Check sheet for the modelled part. Datum: model origin and axes. Units: mm. A direction names the side the tool comes from. Round coordinates to 2 decimals unless told otherwise and drop trailing zeros. Write each loop counter-clockwise with the first axis right and the second up, starting at its lowest first coordinate (ties: lowest second). Pieces come first, ordered by that corner, then holes. Notation, with made-up numbers: (82, 4.5) -> (93, 4.5) arc R19 ccw to (93, 17.5) -> close; hole circle Ø8 at (30.25, 42). An arc over 180 degrees is marked (long way). One line per item, written item: value.
from build123d import *

# Parameters (mm, degrees)
BOSS_EXTRUDE1_DEPTH = 5
SKETCH3_R           = 10.5
CUT_EXTRUDE1_DEPTH  = 1
SKETCH4_R           = 2.5
BOSS_EXTRUDE2_DEPTH = 6
SKETCH5_R           = 1.5
CUT_EXTRUDE2_DEPTH  = 3
CUT_EXTRUDE3_DEPTH  = 1
SKETCH7_R           = 1.25
CUT_EXTRUDE4_DEPTH  = 5
SKETCH8_R           = 2.5
CUT_EXTRUDE5_DEPTH  = 0.5
CUT_EXTRUDE6_DEPTH  = 2
CUT_EXTRUDE7_DEPTH  = 2
SKETCH12_R          = 12.1
BOSS_EXTRUDE3_DEPTH = 15
SKETCH13_R          = 10.4
SKETCH13_R_2        = 2.5
CUT_EXTRUDE8_DEPTH  = 14
SKETCH14_R          = 1.5
CUT_EXTRUDE9_DEPTH  = 5


with BuildPart() as part:
    # Sketch1 → Boss-Extrude1 (new body)
    with BuildSketch(Plane(origin=(0, 0, 0), x_dir=(1, 0, 0), z_dir=(0, 1, 0))):
        with BuildLine():
            Line((-22, -23.004932369), (-22, -33.004932369))
            Line((-22, -33.004932369), (-13.5, -33.004932369))
            Line((-13.5, -33.004932369), (-8.890227771, -30.004932369))
            Line((-8.890227771, -30.004932369), (-7.526591408, -32.100283382))
            ThreePointArc((-7.526591408, -32.100283382), (-3.847417482, -30.904492858), (0, -30.5))
            Line((0, -30.5), (0, 12.5))
            ThreePointArc((0, 12.5), (-7.116131574, 10.276705281), (-11.700861907, 4.397707428))
            Line((-11.700861907, 4.397707428), (-22, -23.004932369))
        make_face()
        with BuildLine():
            ThreePointArc((11.700861907, 4.397707428), (7.116131574, 10.276705281), (0, 12.5))
            Line((0, 12.5), (0, -30.5))
            ThreePointArc((0, -30.5), (3.847417482, -30.904492858), (7.526591408, -32.100283382))
            Line((7.526591408, -32.100283382), (8.890227771, -30.004932369))
            Line((8.890227771, -30.004932369), (13.5, -33.004932369))
            Line((13.5, -33.004932369), (22, -33.004932369))
            Line((22, -33.004932369), (22, -23.004932369))
            Line((22, -23.004932369), (11.700861907, 4.397707428))
        make_face()
    extrude(amount=BOSS_EXTRUDE1_DEPTH)

    # Sketch3 → Cut-Extrude1 (cut)
    with BuildSketch(Plane(origin=(0, 5, 0), x_dir=(1, 0, 0), z_dir=(0, 1, 0))):
        Circle(SKETCH3_R)
    extrude(amount=-CUT_EXTRUDE1_DEPTH, mode=Mode.SUBTRACT)

    # Sketch4 → Boss-Extrude2 (add)
    with BuildSketch(Plane(origin=(0, 4, 0), x_dir=(1, 0, 0), z_dir=(0, 1, 0))):
        Circle(SKETCH4_R)
    extrude(amount=BOSS_EXTRUDE2_DEPTH)

    # Sketch5 → Cut-Extrude2 (cut)
    with BuildSketch(Plane(origin=(0, 10, 0), x_dir=(1, 0, 0), z_dir=(0, 1, 0))):
        Circle(SKETCH5_R)
    extrude(amount=-CUT_EXTRUDE2_DEPTH, mode=Mode.SUBTRACT)

    # Sketch6 → Cut-Extrude3 (cut)
    with BuildSketch(Plane(origin=(0, 5, 0), x_dir=(1, 0, 0), z_dir=(0, 1, 0))):
        with BuildLine():
            Line((-1, -12.209115447), (-1, -26.209115447))
            ThreePointArc((-1, -26.209115447), (-7.874005651, -27.593208423), (-14, -31.004932369))
            Line((-14, -31.004932369), (-20, -31.004932369))
            Line((-20, -31.004932369), (-20, -24.004932369))
            Line((-20, -24.004932369), (-11.96508369, -2.626646587))
            ThreePointArc((-11.96508369, -2.626646587), (-8.060972406, -9.224056801), (-1, -12.209115447))
        make_face()
        with BuildLine():
            Line((20, -24.004932369), (11.96508369, -2.626646587))
            ThreePointArc((11.96508369, -2.626646587), (8.060972406, -9.224056801), (1, -12.209115447))
            Line((1, -12.209115447), (1, -26.209115447))
            ThreePointArc((1, -26.209115447), (7.874005651, -27.593208423), (14, -31.004932369))
            Line((14, -31.004932369), (20, -31.004932369))
            Line((20, -31.004932369), (20, -24.004932369))
        make_face()
    extrude(amount=-CUT_EXTRUDE3_DEPTH, mode=Mode.SUBTRACT)

    # Sketch7 → Cut-Extrude4 (cut, through all)
    with BuildSketch(Plane(origin=(0, 4, 0), x_dir=(1, 0, 0), z_dir=(0, 1, 0))):
        with Locations((-15.5, -26.954932369)):
            Circle(SKETCH7_R)
        with Locations((15.5, -26.954932369)):
            Circle(SKETCH7_R)
    extrude(amount=-CUT_EXTRUDE4_DEPTH, mode=Mode.SUBTRACT)

    # Sketch8 → Cut-Extrude5 (cut)
    with BuildSketch(Plane(origin=(0, 4, 0), x_dir=(1, 0, 0), z_dir=(0, 1, 0))):
        with Locations((-15.5, -26.954932369)):
            Circle(SKETCH8_R)
        with Locations((15.5, -26.954932369)):
            Circle(SKETCH8_R)
    extrude(amount=-CUT_EXTRUDE5_DEPTH, mode=Mode.SUBTRACT)

    # Sketch9 → Cut-Extrude6 (cut)
    with BuildSketch(Plane.XZ):
        with BuildLine():
            Line((20, 33.004932369), (20, 27.004932369))
            ThreePointArc((20, 27.004932369), (0, 18), (-20, 27.004932369))
            Line((-20, 27.004932369), (-20, 33.004932369))
            Line((-20, 33.004932369), (20, 33.004932369))
        make_face()
    extrude(amount=-CUT_EXTRUDE6_DEPTH, mode=Mode.SUBTRACT)

    # Sketch11 → Cut-Extrude7 (cut)
    with BuildSketch(Plane.XZ):
        with BuildLine():
            Line((-20, 23.004932369), (-10.073125454, -3.40723582))
            ThreePointArc((-10.073125454, -3.40723582), (0, -10.633772254), (10.073125454, -3.40723582))
            Line((10.073125454, -3.40723582), (20, 23.004932369))
            Line((20, 23.004932369), (20, 25.529642354))
            ThreePointArc((20, 25.529642354), (0, 17.000016389), (-20, 25.529642354))
            Line((-20, 25.529642354), (-20, 23.004932369))
        make_face()
    extrude(amount=-CUT_EXTRUDE7_DEPTH, mode=Mode.SUBTRACT)

    # Sketch12 → Boss-Extrude3 (add)
    with BuildSketch(Plane.XZ.offset(-2)):
        Circle(SKETCH12_R)
    extrude(amount=BOSS_EXTRUDE3_DEPTH)

    # Sketch13 → Cut-Extrude8 (cut)
    with BuildSketch(Plane.XZ.offset(13)):
        Circle(SKETCH13_R)
        Circle(SKETCH13_R_2, mode=Mode.SUBTRACT)
    extrude(amount=-CUT_EXTRUDE8_DEPTH, mode=Mode.SUBTRACT)

    # Sketch14 → Cut-Extrude9 (cut)
    with BuildSketch(Plane.XZ.offset(13)):
        Circle(SKETCH14_R)
    extrude(amount=-CUT_EXTRUDE9_DEPTH, mode=Mode.SUBTRACT)


solid = part.part
Item 1: Thickness scan on line 1 (X direction, y = 4.75, z = 25); line 2 (Z direction, x = 0, y = -10); line 3 (X direction, y = 8.5, z = 0). Record the ranges inside material, lowest first.
Answer:
line 1: x = -22 to -20, -1 to 1, 20 to 22
line 2: z = -12.1 to -10.4, -2.5 to -1.5, 1.5 to 2.5, 10.4 to 12.1
line 3: x = -2.5 to -1.5, 1.5 to 2.5
Item 2: Mould release check, pull along X, two halves, no side actions. Record for faces 5 (the flat face through (22, 2, 28)), 6 (the flat face through (-19, 3, 33.005)), 7 (the flat face through (0, 2, 15)): pulls with the +X half, pulls with the -X half, needs draft (parallel to the pull), parting line crosses it, or undercut.
Answer:
face 5: pulls with the +X half
face 6: needs draft
face 7: undercut
Item 3: Tool access check on faces 1 (the cylindrical face through (10, 4.5, -3.2)), 2 (the cylindrical face through (0, 1, 18)), 3 (the flat face through (15.936, 0.986, 12.191)), 4 (the flat face through (-8.218, 3.479, 31.038)). Record the directions out of +Z, -Z, +X, -X, +Y, -Y that give a thin tool (end or side, any length) a straight path to the whole face; none if there is none.
Answer:
face 1: +Y
face 2: +Z, -Y
face 3: -Y
face 4: +Z, +Y, -Y
Item 4: Sectioned sample at D-D on z = -5.5. Enter the section's corners in (x, y).
Answer:
outline: (-11.22, 0) -> (-10.78, 0) -> (-10.78, -13) -> (-8.83, -13) -> (-8.83, 1) -> (8.83, 1) -> (8.83, -13) -> (10.78, -13) -> (10.78, 0) -> (11.22, 0) -> (11.22, 5) -> (8.94, 5) -> (8.94, 4) -> (-8.94, 4) -> (-8.94, 5) -> (-11.22, 5) -> close
Item 5: Sectioned sample at C-C on x = -15. Enter the section's corners in (y, z).
Answer:
outline: (0, 4.38) -> (5, 4.38) -> (5, 10.7) -> (4, 10.7) -> (4, 24.51) -> (3.5, 24.51) -> (3.5, 25.81) -> (2, 25.81) -> (2, 22.61) -> (0, 22.61) -> (0, 21.41) -> (2, 21.41) -> (2, 9.7) -> (0, 9.7) -> close; (2, 28.1) -> (3.5, 28.1) -> (3.5, 29.4) -> (4, 29.4) -> (4, 31) -> (5, 31) -> (5, 33) -> (2, 33) -> close
Item 6: Sectioned sample at B-B on y = -11.5. Enter the section's corners in (x, z), and give its area (3 significant figures).
Answer:
outline: circle Ø24.2 at (0, 0); circle Ø5 at (0, 0); hole circle Ø20.8 at (0, 0); hole circle Ø3 at (0, 0)
area: 133 mm^2
Item 7: Sectioned sample at A-A on y = -5.75. Enter the section's corners in (x, z).
Answer:
outline: circle Ø24.2 at (0, 0); circle Ø5 at (0, 0); hole circle Ø20.8 at (0, 0)
Item 8: Depth check by flat-ended pin: P1, Ø1.5, axis at x = 15.5, z = 26.95, coming from the -Y side; P2, Ø4, axis at y = 4.5, z = 12.5, coming from the -X side; P3, Ø4, axis at x = 16.5, z = 26.5, coming from the +Y side; P4, Ø12, axis at x = 2.5, y = 1.5, coming from the +Z side. Enter the tip coordinate at first touch or a pass-through.
Answer:
P1: passes through
P2: stops at x = -18.8
P3: stops at y = 4
P4: stops at z = 32.1
